Job drawing, mm, ordinate dimensions from the low corner. One solid piece. A direction names the side the tool comes from. Round coordinates to 2 decimals unless told otherwise and drop trailing zeros. Write each loop counter-clockwise with the first axis right and the second up, starting at its lowest first coordinate (ties: lowest second). Pieces come first, ordered by that corner, then holes. Notation, with made-up numbers: M 16,66 L 45,66 A11 cw 45,77 Z; hole C 40,-10 d5. An arc over 180 degrees is marked long. One line per item, written item: value. Start each with the question number.
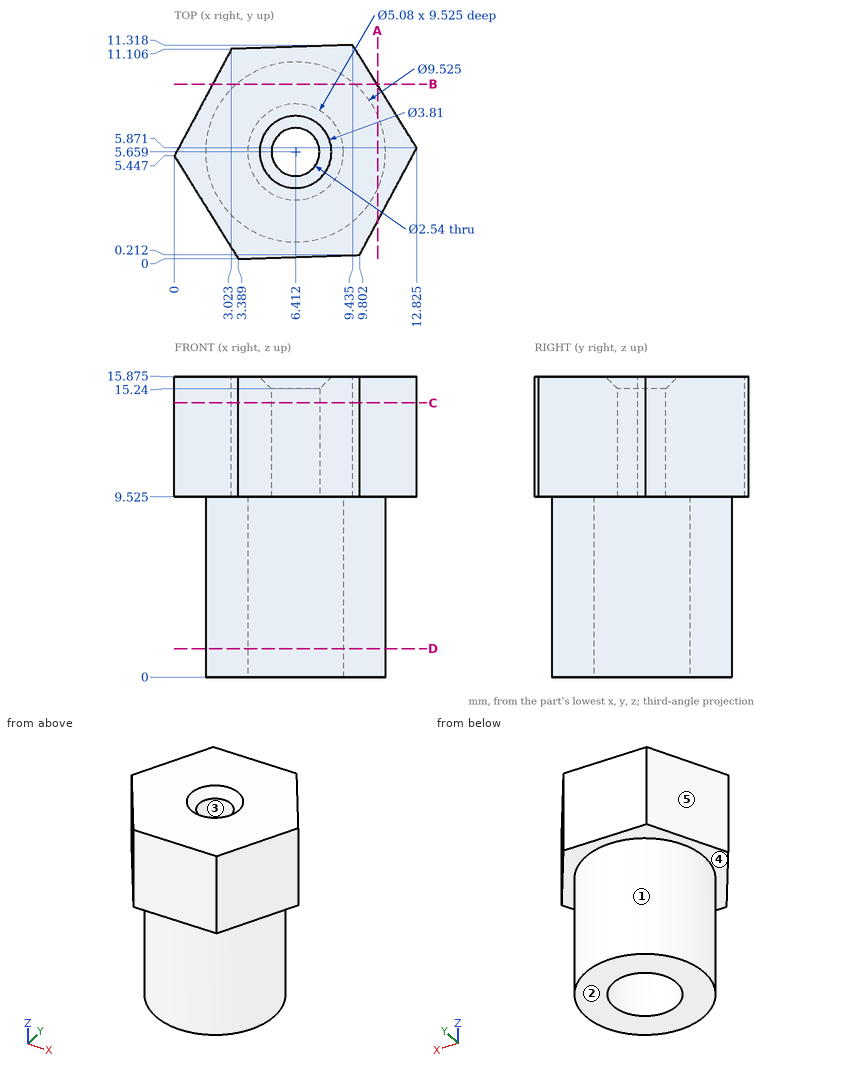
Item 1: Which spindle directions (+Z, -Z, +X, -X, +Y, -Y) get a long thin tool onto all of the face, cutting with end or side? Do the marked faces 4 and 5. Say none if no direction does.
Item 2: Two-plate mould, pull along Y, no slides. Class the marked faces 1, 2 and 3: pulls with the +Y half, pulls with the -Y half, needs draft (parallel to the pull), parting line crosses it, or undercut.
Item 3: Cut at C-C, the plane z = 14.5. Write the cut outline in (x, y) (1 decimal).
Item 4: Drill centre lines: line 1 (X direction, y = 5, z = 9.25) (1 decimal); line 2 (Z direction, x = 11.5, y = 5.5) (1 decimal); line 3 (X direction, y = 7.5, z = 5.5) (1 decimal). Where is each one in solid material? Low to high.
Item 5: Cut at D-D, the plane z = 1.5. Write the cut outline in (x, y) (1 decimal).
Item 6: Drop flat-ended pins along their axis: pin 1 (1.5 mm diameter, centred on y = 8.5, z = 8.5, fed in from +X); pin 2 (1 mm diameter, centred on y = 1.5, z = 3, fed in from +X); pin 3 (5 mm diameter, centred on x = 3.5, z = 3.5, fed in from -Y). Give the stop position or say it passes through.
Item 7: Cut at B-B, the plane y = 9.25. Write the cut outline in (x, z) (1 decimal).
Item 8: Cut at A-A, the plane x = 10.75. Write the cut outline in (y, z) (1 decimal).
Computed values:
1. face 4: -Z
1. face 5: +Z, -Z, -X, +Y
2. face 1: parting line crosses it
2. face 2: needs draft
2. face 3: undercut
3. outline: M 0,5.4 L 3.4,0 L 9.8,0.2 L 12.8,5.9 L 9.4,11.3 L 3,11.1 Z; hole C 6.4,5.7 d2.5
4. line 1: x = 1.7 to 4, 8.9 to 11.1
4. line 2: z = 9.5 to 15.9
4. line 3: x = 2 to 4.7, 8.2 to 10.8
5. outline: C 6.4,5.7 d9.5; hole C 6.4,5.7 d5.1
6. pin 1: stops at x = 10.69
6. pin 2: stops at x = 9.46
6. pin 3: stops at y = 0.91
7. outline: M 2,9.5 L 3.3,9.5 L 3.3,0 L 9.5,0 L 9.5,9.5 L 10.7,9.5 L 10.7,15.9 L 2,15.9 Z
8. outline: M 2,9.5 L 3.7,9.5 L 3.7,0 L 7.6,0 L 7.6,9.5 L 9.2,9.5 L 9.2,15.9 L 2,15.9 Z
